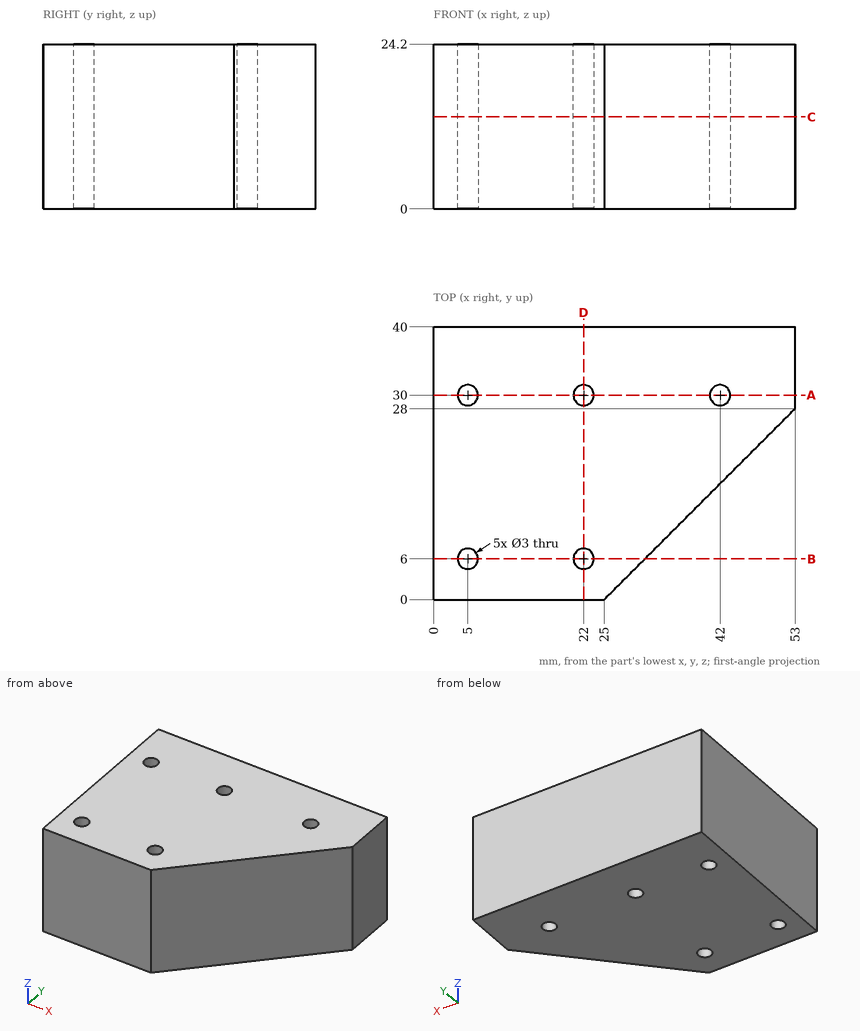
Study the drawing (mm; zero at the part's minimum x, y, z) and answer. Round coordinates to 2 decimals unless told otherwise and drop trailing zeros. Loops run counter-clockwise (first coordinate to the right, second up) from the corner with the lowest first, then second, coordinate; pieces in that order, holes last.
Q1. Find the intervals of material crossed by line 1 (Y direction, x = 22, z = 7); line 2 (Y direction, x = 21, z = 6.25); line 3 (X direction, y = 5, z = 15.5), in increasing order.
Q2. Section C-C, the plane z = 13.5 is taken. Determine the outline of the cut face in (x, y), then the cut area to 3 significant figures.
Q3. Given pin 1 Ø5 at (y, z) = (4.5, 17.5) entering from +X; pin 2 Ø10 at (y, z) = (13.5, 12) entering from +X, each flat-ended and moving along its own axis, determine where each tip first touches the part or whether it passes through.
Q4. Section D-D, the plane x = 22 is taken. Determine the outline of the cut face in (y, z).
Q5. Section B-B, the plane y = 6 is taken. Determine the outline of the cut face in (x, z).
Q6. Section A-A, the plane y = 30 is taken. Determine the outline of the cut face in (x, z).
Completed:
1. line 1: y = 0 to 4.5, 7.5 to 28.5, 31.5 to 40
1. line 2: y = 0 to 4.88, 7.12 to 28.88, 31.12 to 40
1. line 3: x = 0 to 3.88, 6.12 to 20.88, 23.12 to 30
2. outline: (0, 0) - (25, 0) - (53, 28) - (53, 40) - (0, 40) - close; hole circle Ø3 at (5, 6); hole circle Ø3 at (5, 30); hole circle Ø3 at (22, 6); hole circle Ø3 at (22, 30); hole circle Ø3 at (42, 30)
2. area: 1,690 mm2
3. pin 1: stops at x = 32
3. pin 2: stops at x = 43.5
4. outline: (0, 0) - (4.5, 0) - (4.5, 24.2) - (0, 24.2) - close; (7.5, 0) - (28.5, 0) - (28.5, 24.2) - (7.5, 24.2) - close; (31.5, 0) - (40, 0) - (40, 24.2) - (31.5, 24.2) - close
5. outline: (0, 0) - (3.5, 0) - (3.5, 24.2) - (0, 24.2) - close; (6.5, 0) - (20.5, 0) - (20.5, 24.2) - (6.5, 24.2) - close; (23.5, 0) - (31, 0) - (31, 24.2) - (23.5, 24.2) - close
6. outline: (0, 0) - (3.5, 0) - (3.5, 24.2) - (0, 24.2) - close; (6.5, 0) - (20.5, 0) - (20.5, 24.2) - (6.5, 24.2) - close; (23.5, 0) - (40.5, 0) - (40.5, 24.2) - (23.5, 24.2) - close; (43.5, 0) - (53, 0) - (53, 24.2) - (43.5, 24.2) - close
